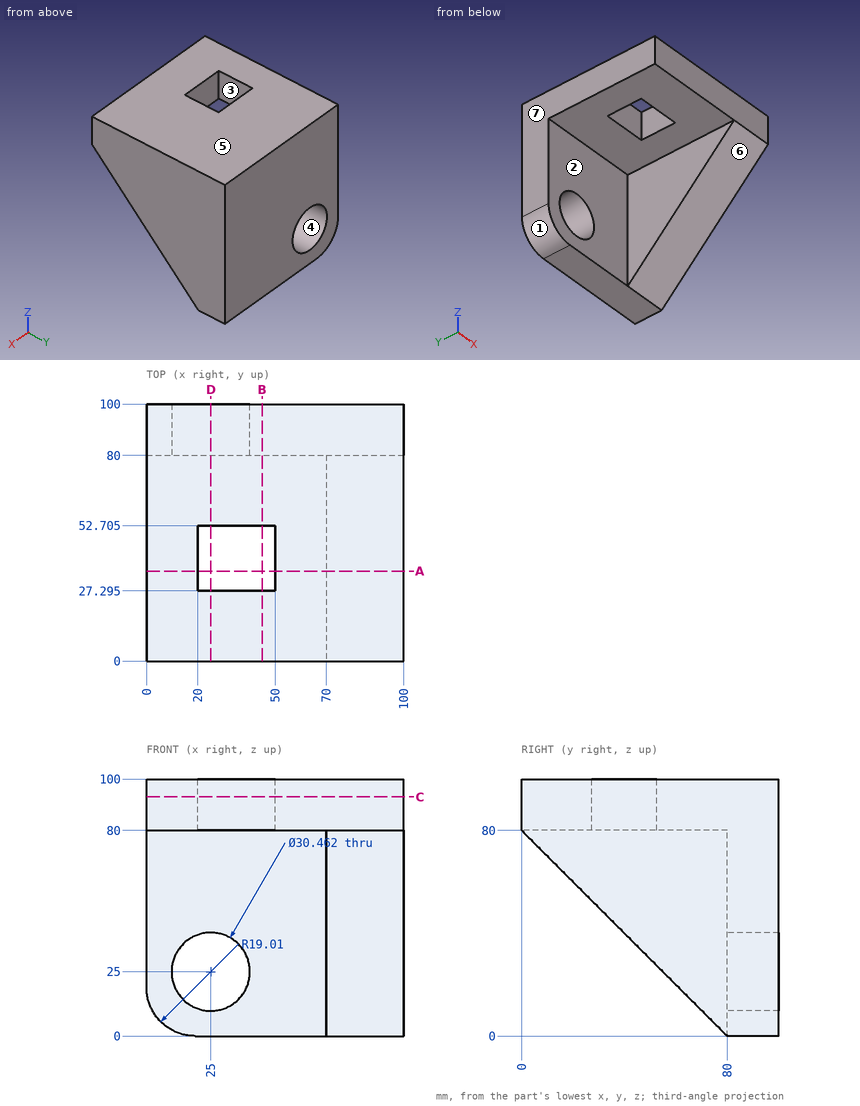
Input: dimensioned drawing with shaded views. Units: mm. Origin: part minimum x, y, z. A direction names the side the tool comes from. Give positions to 0.01 mm unless a question says otherwise; leave off trailing zeros. Write each loop counter-clockwise with the first axis right and the second up, starting at its lowest first coordinate (ties: lowest second). Pieces come first, ordered by that corner, then holes. Notation, with made-up numbers: (34.25, 32.25) - (92.25, 32.25) arc R24 ccw to (92.25, 52.25) - close; hole circle Ø5 at (-24.75, 3.25). An arc over 180 degrees is marked (long way). Write item = value, one per line. Start each with the question number.
1) Draft query along Z for the marked faces 4, 5, 6 and 7. Return one class per face: pulls with the +Z half, pulls with the -Z half, needs draft (parallel to the pull), parting line crosses it, or undercut.
2) Cut plane A-A (y = 35). Return loops of the section in (x, z).
3) Material intervals for L1, parallel to Z at x = 25, y = 92; L2, parallel to Y at x = 48, z = 84.5 (1 decimal); L3, parallel to Y at x = 19, z = 71, sorted ascending. Write a range as [from, to].
4) Cut plane C-C (z = 93). Return loops of the section in (x, y) (1 decimal), and give its area (3 significant figures).
5) Reachability of the marked faces 1, 2 and 3 from +Z, -Z, +X, -X, +Y, -Y: full face, straight path, thin tool, end or side. Return the list, or none.
6) Cut plane D-D (x = 25). Return loops of the section in (y, z) (1 decimal).
7) Pin query (flat end, axial travel): pin 1 (8 mm diameter, centred on y = 38.5, z = 57.5, fed in from -X); pin 2 (5 mm diameter, centred on x = 58.5, y = 29, fed in from -Z); pin 3 (12 mm diameter, centred on x = 67.5, z = 39.5, fed in from -Y) (1 decimal). Return the tip coordinate at first contact, or that it passes through.
8) Cut plane B-B (x = 45). Return loops of the section in (y, z) (1 decimal), and give its area (3 significant figures).
Answers follow:
q1.face_4 = undercut
q1.face_5 = pulls with the +Z half
q1.face_6 = pulls with the -Z half
q1.face_7 = needs draft
q2.outline = (0, 80) - (20, 80) - (20, 100) - (0, 100) - close; (50, 80) - (70, 80) - (70, 45) - (100, 45) - (100, 100) - (50, 100) - close
q3.L1 = [0, 9.77], [40.23, 100]
q3.L2 = [0, 27.3], [52.7, 100]
q3.L3 = [80, 100]
q4.outline = (0, 0) - (100, 0) - (100, 100) - (0, 100) - close; hole (20, 27.3) - (50, 27.3) - (50, 52.7) - (20, 52.7) - close
q4.area = 9,240 mm^2
q5.face_1 = -Z, -X, +Y, -Y
q5.face_2 = -Z, -X, -Y
q5.face_3 = +Z, -Z
q6.outline = (0, 80) - (27.3, 80) - (27.3, 100) - (0, 100) - close; (52.7, 80) - (80, 80) - (80, 40.2) - (100, 40.2) - (100, 100) - (52.7, 100) - close; (80, 0) - (100, 0) - (100, 9.8) - (80, 9.8) - close
q7.pin_1 = 70
q7.pin_2 = 80
q7.pin_3 = 35
q8.outline = (0, 80) - (27.3, 80) - (27.3, 100) - (0, 100) - close; (52.7, 80) - (80, 80) - (80, 0) - (100, 0) - (100, 100) - (52.7, 100) - close
q8.area = 3,090 mm^2
